from build123d import *

# Parameters (mm, degrees)
SKETCH1_W           = 510
SKETCH1_H           = 540
BOSS_EXTRUDE1_DEPTH = 3
CUT_EXTRUDE2_REACH  = 373.395
SKETCH3_W           = 400
SKETCH3_H           = 120


with BuildPart() as part:
    # Sketch1 → Boss-Extrude1 (new body)
    with BuildSketch(Plane.XY):
        Rectangle(SKETCH1_W, SKETCH1_H)
    extrude(amount=BOSS_EXTRUDE1_DEPTH)

    # Sketch3 → Cut-Extrude2 (cut, up to next)
    with BuildSketch(Plane.XY.offset(3), mode=Mode.PRIVATE) as cut_extrude2_sk1:
        Rectangle(SKETCH3_W, SKETCH3_H)
    cut_extrude2_tool1 = extrude(cut_extrude2_sk1.sketch, amount=-CUT_EXTRUDE2_REACH, mode=Mode.PRIVATE) & part.part
    add(cut_extrude2_tool1.solids().sort_by_distance((0, 0, 3))[0], mode=Mode.SUBTRACT)


solid = part.part
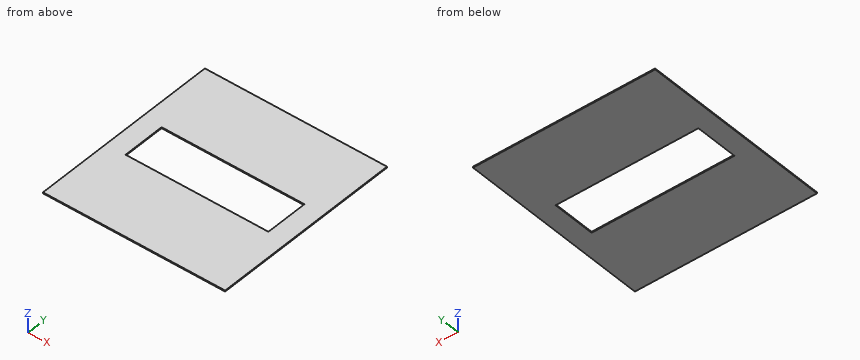
Read the model definition and answer for the solid it produces. Units are mm, in the model's axes. Round coordinates to 2 decimals unless told otherwise and drop trailing zeros. Write each loop counter-clockwise with the first axis right and the second up, starting at its lowest first coordinate (ties: lowest second). Pieces come first, ordered by that corner, then holes.
1. The part is cut by section B-B, the plane y = 3. Determine the outline of the cut face in (x, z), then the cut area to 3 significant figures.
2. The part is cut by section C-C, the plane z = 0.7. Determine the outline of the cut face in (x, y).
3. The part is cut by section A-A, the plane x = 175. Determine the outline of the cut face in (y, z), then the cut area to 3 significant figures.
4. Straight lines are drawn through the part: L1, parallel to Y at x = -197, z = 0.4; L2, parallel to X at y = 0, z = 0.4. For each, find the intervals that lie inside material, in ascending order.
Values:
1. outline: (-255, 0) - (-200, 0) - (-200, 3) - (-255, 3) - close; (200, 0) - (255, 0) - (255, 3) - (200, 3) - close
1. area: 330 mm2
2. outline: (-255, -270) - (255, -270) - (255, 270) - (-255, 270) - close; hole (-200, -60) - (200, -60) - (200, 60) - (-200, 60) - close
3. outline: (-270, 0) - (-60, 0) - (-60, 3) - (-270, 3) - close; (60, 0) - (270, 0) - (270, 3) - (60, 3) - close
3. area: 1,260 mm2
4. L1: y = -270 to -60, 60 to 270
4. L2: x = -255 to -200, 200 to 255
